Can you work these out from the model? Positions are in its coordinate system, mm. Face numbers are marked on the shaded views. A direction names the side the tool comes from. Round coordinates to 2 decimals unless told otherwise and drop trailing zeros. Write each loop counter-clockwise with the first axis right and the second up, starting at its lowest first coordinate (ties: lowest second). Pieces come first, ordered by that corner, then holes.
Q1. If we section it at B-B (z = 0.5): Please give me the cut outline in (x, y), plus the area to 3 significant figures.
Q2. Please list where these lines run through material, in increasing order: line 1 along Z through (x, y) = (5, -21); line 2 along X through (y, z) = (-18.84, -7.5); line 3 along X through (y, z) = (-18.84, 10.5).
Q3. If we section it at C-C (x = 22): Please give me the cut outline in (y, z), plus the area to 3 significant figures.
Q4. If we section it at D-D (z = -7.5): Please give me the cut outline in (x, y), plus the area to 3 significant figures.
Q5. If we section it at A-A (y = -22.84): Please give me the cut outline in (x, z), plus the area to 4 significant figures.
Q6. We'd pull the mould along Y, two halves only. Please class the marked faces 6, 7 and 8: +Y half, -Y half, draft (parallel to the pull), parting line (faces both ways), or undercut.
Q7. For the marked faces 1, 2, 3, 4 and 5, which set-ups out of +Z, -Z, +X, -X, +Y, -Y let a thin tool reach every point of the face, with its end or its side?
Q8. I'm going to push flat-ended pins straight in: pin 1 Ø1 at (y, z) = (-32, 10) entering from -X; pin 2 Ø12.5 at (x, z) = (-31, 2.5) entering from +Y; pin 3 Ø18 at (x, y) = (-31.47, -22.84) entering from -Z; pin 4 Ø4 at (x, z) = (-20, -1.5) entering from -Y. Where does each tip first touch, or does it pass through?
from build123d import *

# Parameters (mm, degrees)
SKETCH1_W           = 27
SKETCH1_H           = 33
SKETCH1_R           = 7
SKETCH1_R_2         = 5
BOSS_EXTRUDE1_DEPTH = 12.5
CUT_EXTRUDE1_START  = 4.5
SKETCH1_3_W         = 27
SKETCH1_3_H         = 33
SKETCH1_3_R         = 7
CUT_EXTRUDE1_DEPTH  = 8
CHAMFER1_SIZE       = 5
CUT_EXTRUDE2_DEPTH  = 5.5


with BuildPart() as part:
    # Sketch1 → Boss-Extrude1 (new, symmetric)
    # profile 1 of 2: a face of its own
    with BuildSketch(Plane.XY):
        with Locations((-33.967633793, -25.34)):
            Rectangle(SKETCH1_W, SKETCH1_H)
        with Locations((-31.467633793, -22.84)):
            Circle(SKETCH1_R, mode=Mode.SUBTRACT)
    # profile 2 of 2: a face of its own
    with BuildSketch(Plane.XY):
        with BuildLine():
            Line((37.532366207, -3.84), (25.532366207, -3.84))
            Line((25.532366207, -3.84), (15.532366207, -3.84))
            ThreePointArc((15.532366207, -3.84), (6.522255442, -14.610276655), (-7.511545005, -14.127161486))
            Line((-7.511545005, -14.127161486), (-17.455249537, -8.84))
            Line((-17.455249537, -8.84), (-20.467633793, -8.84))
            Line((-20.467633793, -8.84), (-20.467633793, -41.84))
            Line((-20.467633793, -41.84), (-17.965724565, -41.84))
            ThreePointArc((-17.965724565, -41.84), (-12.096906214, -43.743274047), (-8.462081793, -48.728605767))
            ThreePointArc((-8.462081793, -48.728605767), (-5.535546312, -55.58874428), (-1.467633793, -61.84))
            Line((-1.467633793, -61.84), (11.532366207, -61.84))
            Line((11.532366207, -61.84), (37.532366207, -28.84))
            Line((37.532366207, -28.84), (37.532366207, -3.84))
        make_face()
        with Locations((25.532366207, -18.84)):
            Circle(SKETCH1_R_2, mode=Mode.SUBTRACT)
    extrude(amount=BOSS_EXTRUDE1_DEPTH, both=True)

    # Sketch1_3 → Cut-Extrude1 (cut)
    with BuildSketch(Plane.XY.offset(CUT_EXTRUDE1_START)):
        with Locations((-33.967633793, -25.34)):
            Rectangle(SKETCH1_3_W, SKETCH1_3_H)
        with Locations((-31.467633793, -22.84)):
            Circle(SKETCH1_3_R, mode=Mode.SUBTRACT)
    extrude(amount=CUT_EXTRUDE1_DEPTH, mode=Mode.SUBTRACT)

    # Chamfer1
    chamfer1_edges = [part.edges().sort_by_distance(p)[0] for p in [
        (37.532366207, -3.84, 0),
        (-47.467633793, -41.84, -4),
        (-47.467633793, -8.84, -4),
    ]]
    chamfer(chamfer1_edges, length=CHAMFER1_SIZE)

    # Sketch4 → Cut-Extrude2 (cut, symmetric)
    with BuildSketch(Plane.XY):
        with BuildLine():
            Line((37.532366207, -8.84), (37.532366207, -28.84))
            Line((37.532366207, -28.84), (28.205719919, -40.677666444))
            ThreePointArc((28.205719919, -40.677666444), (11.699513519, -31.708687123), (1.506567213, -15.928912557))
            ThreePointArc((1.506567213, -15.928912557), (10.445897028, -12.1195394), (15.532366207, -3.84))
            Line((15.532366207, -3.84), (32.532366207, -3.84))
            Line((32.532366207, -3.84), (37.532366207, -8.84))
        make_face()
    extrude(amount=CUT_EXTRUDE2_DEPTH, both=True, mode=Mode.SUBTRACT)


solid = part.part
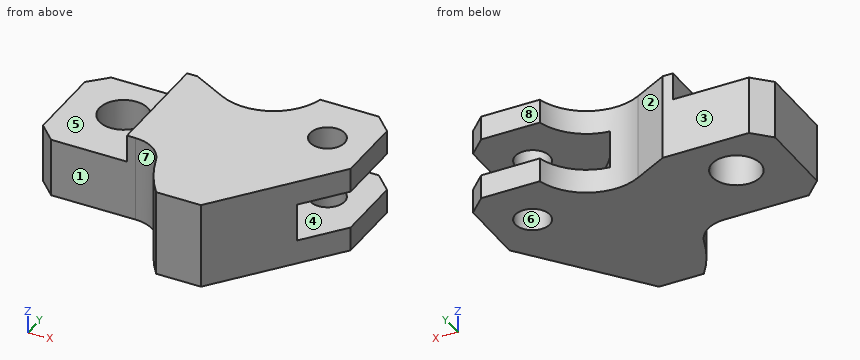
A:
1. outline: (-47.47, -36.84) - (-42.47, -41.84) - (-17.97, -41.84) arc R10 cw to (-8.46, -48.73) arc R43 ccw to (-1.47, -61.84) - (11.53, -61.84) - (28.21, -40.68) arc R38 cw to (1.51, -15.93) arc R16 cw to (-7.51, -14.13) - (-17.46, -8.84) - (-42.47, -8.84) - (-47.47, -13.84) - close; hole circle Ø14 at (-31.47, -22.84)
1. area: 2,130 mm2
2. line 1: z = -12.5 to -5.5, 5.5 to 12.5
2. line 2: x = -47.47 to -37.21, -25.72 to 20.53, 30.53 to 37.53
2. line 3: x = -20.47 to 20.53, 30.53 to 37.53
3. outline: (-48.55, -12.5) - (-22.38, -12.5) - (-22.38, -5.5) - (-38.52, -5.5) - (-38.52, 5.5) - (-22.38, 5.5) - (-22.38, 12.5) - (-48.55, 12.5) - close; (-15.3, -12.5) - (-3.84, -12.5) - (-3.84, -5.5) - (-15.3, -5.5) - close; (-15.3, 5.5) - (-3.84, 5.5) - (-3.84, 12.5) - (-15.3, 12.5) - close
3. area: 637 mm2
4. outline: (-47.47, -36.84) - (-42.47, -41.84) - (-17.97, -41.84) arc R10 cw to (-8.46, -48.73) arc R43 ccw to (-1.47, -61.84) - (11.53, -61.84) - (37.53, -28.84) - (37.53, -8.84) - (32.53, -3.84) - (15.53, -3.84) arc R16 cw to (-7.51, -14.13) - (-17.46, -8.84) - (-42.47, -8.84) - (-47.47, -13.84) - close; hole circle Ø14 at (-31.47, -22.84); hole circle Ø10 at (25.53, -18.84)
4. area: 2,980 mm2
5. outline: (-47.47, -12.5) - (-38.47, -12.5) - (-38.47, 4.5) - (-47.47, 4.5) - close; (-24.47, -12.5) - (22.53, -12.5) - (22.53, -5.5) - (4.62, -5.5) - (4.62, 5.5) - (22.53, 5.5) - (22.53, 12.5) - (-20.47, 12.5) - (-20.47, 4.5) - (-24.47, 4.5) - close; (28.53, -12.5) - (37.53, -12.5) - (37.53, -5.5) - (28.53, -5.5) - close; (28.53, 5.5) - (37.53, 5.5) - (37.53, 12.5) - (28.53, 12.5) - close
5. area: 1,225 mm2
6. face 6: undercut
6. face 7: -Y half
6. face 8: +Y half
7. face 1: +Z, -Z, -X, -Y
7. face 2: +Z, -Z, +Y
7. face 3: +Z, -Z, -X, +Y
7. face 4: +X, +Y
7. face 5: +Z, -X, +Y, -Y
8. pin 1: stops at x = -20.47
8. pin 2: stops at y = -8.84
8. pin 3: stops at z = -12.5
8. pin 4: stops at y = -41.84
